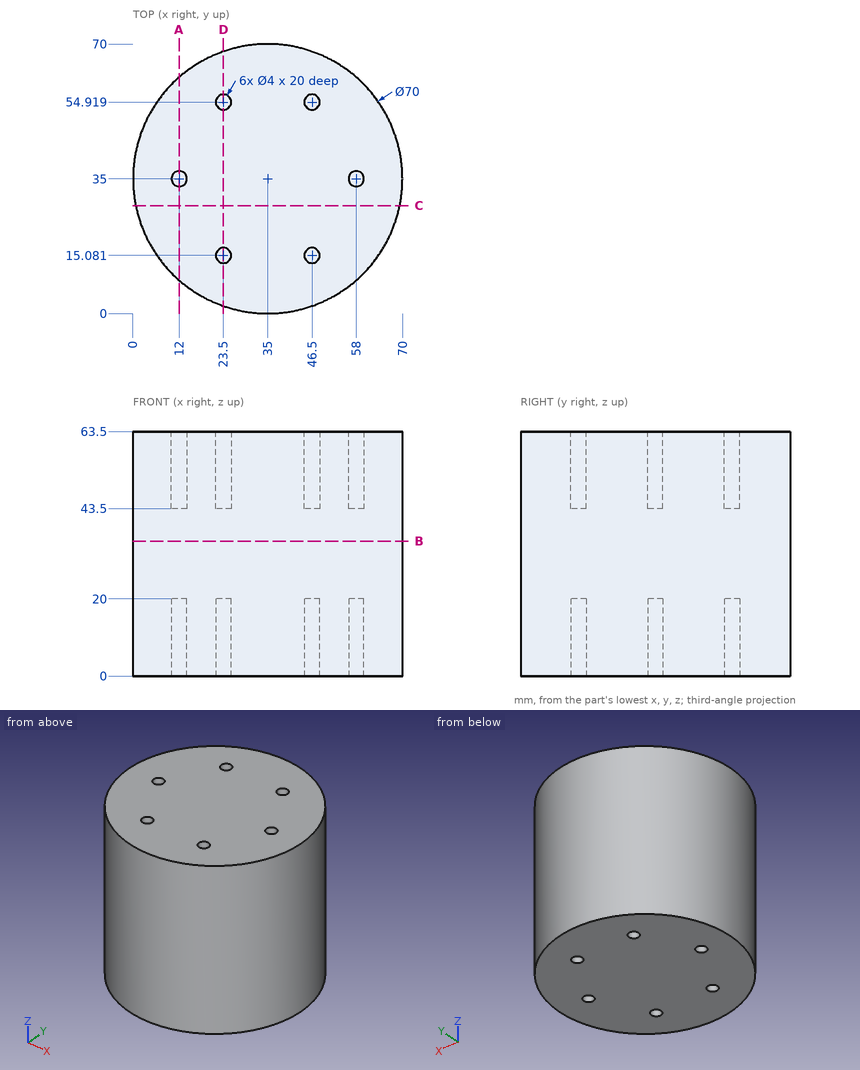
Design review of the part shown in the three views and the two pictorial views. Dimensions are in mm from the part's minimum x, y and z. Coordinates: 2 decimals unless noted, no trailing zeros. Loops run counter-clockwise (first coordinate to the right, second up) from the corner with the lowest first, then second, coordinate; pieces in that order, holes last.
(1) Insertion check: P1, Ø2, axis at x = 57.5, y = 34.5, coming from the -Z side; P2, Ø6, axis at y = 44, z = 21, coming from the -X side; P3, Ø3, axis at x = 23.5, y = 54.92, coming from the +Z side. Each pin has a flat end and moves straight along its axis. Give the tip position at first contact, or say it passes through.
Determined:
P1: stops at z = 20
P2: stops at x = 0.52
P3: stops at z = 43.5
(2) Consider section A-A, the plane x = 12. Give the boundary of the cut face in (y, z), plus the area to 3 significant figures.
Determined:
outline: (8.62, 0) - (33, 0) - (33, 20) - (37, 20) - (37, 0) - (61.38, 0) - (61.38, 63.5) - (37, 63.5) - (37, 43.5) - (33, 43.5) - (33, 63.5) - (8.62, 63.5) - close
area: 3,190 mm2
(3) Consider section C-C, the plane y = 28. Give the boundary of the cut face in (x, z).
Determined:
outline: (0.71, 0) - (69.29, 0) - (69.29, 63.5) - (0.71, 63.5) - close
(4) Wall thickness on L1, parallel to Y at x = 46.5, z = 53.75; L2, parallel to Y at x = 23, z = 48 (1 decimal); L3, parallel to Y at x = 7, z = 42: over which ranges is each line inside the solid? List them lowest first.
Determined:
L1: y = 1.94 to 13.08, 17.08 to 52.92, 56.92 to 68.06
L2: y = 2.1 to 13.1, 17 to 53, 56.9 to 67.9
L3: y = 14 to 56
(5) Consider section D-D, the plane x = 23.5. Give the boundary of the cut face in (y, z).
Determined:
outline: (1.94, 0) - (13.08, 0) - (13.08, 20) - (17.08, 20) - (17.08, 0) - (52.92, 0) - (52.92, 20) - (56.92, 20) - (56.92, 0) - (68.06, 0) - (68.06, 63.5) - (56.92, 63.5) - (56.92, 43.5) - (52.92, 43.5) - (52.92, 63.5) - (17.08, 63.5) - (17.08, 43.5) - (13.08, 43.5) - (13.08, 63.5) - (1.94, 63.5) - close
(6) Consider section B-B, the plane z = 35. Give the boundary of the cut face in (x, y).
Determined:
outline: circle Ø70 at (35, 35)
